from build123d import *

# Parameters (mm, degrees)
EXTRUDE1_DEPTH  = 200
FILLET1_R       = 0.25
LPATTERN1_COUNT = 6
LPATTERN1_PITCH = 38.4
LPATTERN2_COUNT = 6
LPATTERN2_PITCH = 38.4


with BuildPart() as part:
    # Sketch1 → Extrude1 (new body)
    with BuildSketch(Plane.XY):
        Polygon((0, 0), (0, 15), (-15, 15), (-15, 14), (-1, 14), (-1, 0), align=None)
    extrude(amount=EXTRUDE1_DEPTH)

    # Fillet1
    fillet1_edges = [part.edges().sort_by_distance(p)[0] for p in [
        (-15, 14, 100),
        (-15, 15, 100),
        (0, 15, 100),
        (0, 0, 100),
        (-1, 0, 100),
    ]]
    fillet(fillet1_edges, radius=FILLET1_R)

    # Sketch3 → CSK for M3 Countersunk Flat Head Screw1 (revolve, cut)
    with BuildSketch(Plane(origin=(0, 6.5, 4), x_dir=(0, 0, -1), z_dir=(0, 1, 0))):
        Polygon((0, 0), (0, 1.001), (1.7, 1.001), (1.7, 1.45), (3.15, 0), align=None)
    csk_for_m3_countersunk_flat_head_screw1 = revolve(axis=Axis((6.35, 6.5, 4), (-1, 0, 0)), mode=Mode.SUBTRACT)

    # LPattern1: CSK for M3 Countersunk Flat Head Screw1 ×6
    with Locations(*[(0, 0, i * LPATTERN1_PITCH) for i in range(1, LPATTERN1_COUNT)]):
        add(csk_for_m3_countersunk_flat_head_screw1, mode=Mode.SUBTRACT)

    # Sketch5 → CSK for M3 Countersunk Flat Head Screw2 (revolve, cut)
    with BuildSketch(Plane(origin=(-8.5, 15, 4), x_dir=(0, 0, 1), z_dir=(1, 0, 0))):
        Polygon((0, 0), (0, 1.001), (1.7, 1.001), (1.7, 1.45), (3.15, 0), align=None)
    csk_for_m3_countersunk_flat_head_screw2 = revolve(axis=Axis((-8.5, 21.35, 4), (0, -1, 0)), mode=Mode.SUBTRACT)

    # LPattern2: CSK for M3 Countersunk Flat Head Screw2 ×6
    with Locations(*[(0, 0, i * LPATTERN2_PITCH) for i in range(1, LPATTERN2_COUNT)]):
        add(csk_for_m3_countersunk_flat_head_screw2, mode=Mode.SUBTRACT)


solid = part.part
Geometry: final body of the model. Coordinates: model frame, mm. A direction names the side the tool comes from. Coordinates: 2 decimals unless noted, no trailing zeros. Order: outer loops, then holes, each group sorted by start corner. A loop starts at its lowest first (then second) coordinate and runs counter-clockwise, first axis right, second up.
(1) Access query for faces 1 (the face through (-4.2, 14.2, 200)), 2 (the face through (-1, 7, 99)). Directions: +Z, -Z, +X, -X, +Y, -Y. A direction counts if a zero-diameter tool reaches every point of the face in a straight line with its end or side. Return the directions, or none.
(2) Section query A-A (y = 6.5). Return the cut outline in (x, z).
(3) Section query C-C (z = 196). Return the cut outline in (x, y), plus the area to 3 significant figures.
(4) Section query D-D (z = 69). Return the cut outline in (x, y).
(5) First-contact query: pin 1 (5 mm diameter, centred on y = 8, z = 171.5, fed in from -X); pin 2 (5 mm diameter, centred on x = -8.5, y = 13, fed in from -Z); pin 3 (2 mm diameter, centred on y = 7, z = 120.5, fed in from +X). Flat tips, straight axial feed; report the tip coordinate or a pass-through.
(6) Material intervals for probe 1 along Y at (x, z) = (-4, 148.5); probe 2 along X at (y, z) = (3, 27), sorted ascending.
(7) Section query B-B (x = -8.5). Return the cut outline in (y, z), plus the area to 3 significant figures.
Solution:
1. face 1: +Z, +X, -X, +Y, -Y
1. face 2: +Z, -Z, -X, -Y
2. outline: (-1, 0) - (0, 0) - (0, 0.85) - (-1, 1.85) - close; (-1, 6.15) - (0, 7.15) - (0, 39.25) - (-1, 40.25) - close; (-1, 44.55) - (0, 45.55) - (0, 77.65) - (-1, 78.65) - close; (-1, 82.95) - (0, 83.95) - (0, 116.05) - (-1, 117.05) - close; (-1, 121.35) - (0, 122.35) - (0, 154.45) - (-1, 155.45) - close; (-1, 159.75) - (0, 160.75) - (0, 192.85) - (-1, 193.85) - close; (-1, 198.15) - (0, 199.15) - (0, 200) - (-1, 200) - close
3. outline: (-15, 14.25) arc R0.25 ccw to (-14.75, 14) - (-10.65, 14) - (-11.65, 15) - (-14.75, 15) arc R0.25 ccw to (-15, 14.75) - close; (-6.35, 14) - (-1, 14) - (-1, 8.65) - (0, 9.65) - (0, 14.75) arc R0.25 ccw to (-0.25, 15) - (-5.35, 15) - close; (-1, 0.25) arc R0.25 ccw to (-0.75, 0) - (-0.25, 0) arc R0.25 ccw to (0, 0.25) - (0, 3.35) - (-1, 4.35) - close
3. area: 18.3 mm2
4. outline: (-15, 14.25) arc R0.25 ccw to (-14.75, 14) - (-1, 14) - (-1, 0.25) arc R0.25 ccw to (-0.75, 0) - (-0.25, 0) arc R0.25 ccw to (0, 0.25) - (0, 14.75) arc R0.25 ccw to (-0.25, 15) - (-14.75, 15) arc R0.25 ccw to (-15, 14.75) - close
5. pin 1: stops at x = -1
5. pin 2: stops at z = 0
5. pin 3: stops at x = -0.76
6. probe 1: y = 14 to 15
6. probe 2: x = -1 to 0
7. outline: (14, 0) - (15, 0) - (15, 0.85) - (14, 1.85) - close; (14, 6.15) - (15, 7.15) - (15, 39.25) - (14, 40.25) - close; (14, 44.55) - (15, 45.55) - (15, 77.65) - (14, 78.65) - close; (14, 82.95) - (15, 83.95) - (15, 116.05) - (14, 117.05) - close; (14, 121.35) - (15, 122.35) - (15, 154.45) - (14, 155.45) - close; (14, 159.75) - (15, 160.75) - (15, 192.85) - (14, 193.85) - close; (14, 198.15) - (15, 199.15) - (15, 200) - (14, 200) - close
7. area: 168 mm2
